from build123d import *

# Parameters (mm, degrees)
SKETCH001_W     = 143.571686
SKETCH001_H     = 55
PAD001_DEPTH    = 60
SKETCH_R        = 15
PAD_DEPTH       = 42.5
SKETCH002_W     = 45
SKETCH002_H     = 180
PAD002_DEPTH    = 10
SKETCH003_R     = 25
POCKET_DEPTH    = 10
SKETCH004_R     = 10
POCKET001_DEPTH = 25.001


with BuildPart() as pad001:
    # Sketch001 → Pad001 (new body)
    with BuildSketch(Plane(origin=(0, -50, 0), x_dir=(0, 0, -1), z_dir=(0, -1, 0))):
        with Locations((2.390221, 0)):
            Rectangle(SKETCH001_W, SKETCH001_H)
    extrude(amount=PAD001_DEPTH)


with BuildPart() as pocket001:
    # Sketch → Pad (new body, symmetric)
    with BuildSketch(Plane.YZ):
        with BuildLine():
            Line((0, -45), (0, 135))
            Line((0, 135), (-25, 135))
            Line((-25, 135), (-25, 45))
            Line((-25, 45), (-78.708345, 28.708269))
            ThreePointArc((-78.708345, 28.708269), (-100, 2e-06), (-78.708348, -28.708268))
            Line((-78.708348, -28.708268), (-25, -45))
            Line((0, -45), (-25, -45))
        make_face()
        with Locations((-70, 0)):
            Circle(SKETCH_R, mode=Mode.SUBTRACT)
    extrude(amount=PAD_DEPTH, both=True)

    # Cut: cut Pad001
    add(pad001.part, mode=Mode.SUBTRACT)

    # Sketch002 → Pad002 (new body)
    with BuildSketch(Plane(origin=(0, 0, 0), x_dir=(-1, 0, 0), z_dir=(0, 1, 0))):
        with Locations((0, 45)):
            Rectangle(SKETCH002_W, SKETCH002_H)
    extrude(amount=PAD002_DEPTH)

    # Sketch003 → Pocket (cut)
    with BuildSketch(Plane.XZ.offset(25)):
        with Locations((0, 93)):
            Circle(SKETCH003_R)
    extrude(amount=-POCKET_DEPTH, mode=Mode.SUBTRACT)

    # Sketch004 → Pocket001 (cut, through all)
    with BuildSketch(Plane.XZ.offset(15)):
        with Locations((0, 93)):
            Circle(SKETCH004_R)
    extrude(amount=-POCKET001_DEPTH, mode=Mode.SUBTRACT)


solid = pocket001.part
Check sheet for the modelled part. Datum: model origin and axes. Units: mm. A direction names the side the tool comes from. Give positions to 0.01 mm unless a question says otherwise; leave off trailing zeros. Write each loop counter-clockwise with the first axis right and the second up, starting at its lowest first coordinate (ties: lowest second). Pieces come first, ordered by that corner, then holes. Notation, with made-up numbers: (76, 89) -> (120, 89) arc R28 cw to (120, 123) -> close; hole circle Ø9 at (-24, 37.25). An arc over 180 degrees is marked (long way). Use one line per item in the form item = value. Start each with the question number.
1. Go/stop test with flat-tipped pins: P1, Ø8, axis at y = 7, z = 27.5, coming from the -X side; P2, Ø6, axis at x = 19, z = 21.5, coming from the -Y side; P3, Ø6, axis at x = 31.5, y = -77.5, coming from the -Z side. Record where each tip stops, or that it passes through.
2. Mould release check, pull along X, two halves, no side actions. Record for faces 1 (the flat face through (27.5, -86, 1)), 2 (the flat face through (-27.5, -86, 1)), 3 (the flat face through (-22.5, 5, 44)), 4 (the flat face through (1, -11, -45)): pulls with the +X half, pulls with the -X half, needs draft (parallel to the pull), parting line crosses it, or undercut.
3. Section check A-A (z = 93). Record the cut outline in (x, y), and give its area (4 significant figures).
4. Section check D-D (x = -33). Record the cut outline in (y, z), and give its area (3 significant figures).
5. Section check C-C (z = 0). Record the cut outline in (x, y), and give its area (3 significant figures).
6. Section check B-B (x = 0). Record the cut outline in (y, z), and give its area (3 significant figures).
7. Thickness scan on line 1 along Z through (x, y) = (0, 1); line 2 along Y through (x, z) = (-18, 86); line 3 along Y through (x, z) = (14.5, 13). Record the ranges inside material, lowest first. Write a range as from..to.
8. Access from +Z, -Z, +X, -X, +Y, -Y to the whole of each face (thin tool, end or side, straight path). Record for faces 5 (the flat face through (0, -50, 1)), 6 (the flat face through (22.5, 5, 44)), 7 (the cylindrical face through (-5.42, -20.07, 68.594)), 8 (the flat face through (-18, -25, 111)).
Conclusion:
q1.P1 = -22.5
q1.P2 = -50
q1.P3 = -29.98
q2.face_1 = undercut
q2.face_2 = undercut
q2.face_3 = pulls with the -X half
q2.face_4 = needs draft
q3.outline = (-42.5, -25) -> (-25, -25) -> (-25, -15) -> (-10, -15) -> (-10, 10) -> (-22.5, 10) -> (-22.5, 0) -> (-42.5, 0) -> close; (10, -15) -> (25, -15) -> (25, -25) -> (42.5, -25) -> (42.5, 0) -> (22.5, 0) -> (22.5, 10) -> (10, 10) -> close
q3.area = 1,575 mm²
q4.outline = (-78.71, -28.71) -> (-25, -45) -> (0, -45) -> (0, 135) -> (-25, 135) -> (-25, 45) -> (-78.71, 28.71) arc R30 ccw to start; hole circle Ø30 at (-70, 0)
q4.area = 8,650 mm²
q5.outline = (-42.5, -100) -> (-27.5, -100) -> (-27.5, -85) -> (-42.5, -85) -> close; (-42.5, -55) -> (-27.5, -55) -> (-27.5, -50) -> (27.5, -50) -> (27.5, -55) -> (42.5, -55) -> (42.5, 0) -> (22.5, 0) -> (22.5, 10) -> (-22.5, 10) -> (-22.5, 0) -> (-42.5, 0) -> close; (27.5, -100) -> (42.5, -100) -> (42.5, -85) -> (27.5, -85) -> close
q5.area = 5,300 mm²
q6.outline = (-50, -37.42) -> (-25, -45) -> (10, -45) -> (10, 83) -> (-15, 83) -> (-15, 68) -> (-25, 68) -> (-25, 45) -> (-50, 37.42) -> close; (-25, 118) -> (-15, 118) -> (-15, 103) -> (10, 103) -> (10, 135) -> (-25, 135) -> close
q6.area = 7,360 mm²
q7.line_1 = -45..83, 103..135
q7.line_2 = -15..10
q7.line_3 = -50..10
q8.face_5 = +Z, -Z, -Y
q8.face_6 = +Z, -Z, +X, +Y
q8.face_7 = -Y
q8.face_8 = +Z, +X, -X, -Y
